Input: dimensioned drawing with shaded views. Units: mm. Origin: part minimum x, y, z. A direction names the side the tool comes from. Round coordinates to 2 decimals unless told otherwise and drop trailing zeros. Loops run counter-clockwise (first coordinate to the right, second up) from the corner with the lowest first, then second, coordinate; pieces in that order, holes last. Notation, with made-up numbers: M 50.5,59.5 L 106.5,59.5 A21 ccw 106.5,69.5 Z; hole C 2,41 d4. An arc over 180 degrees is marked long. One line per item, written item: value.
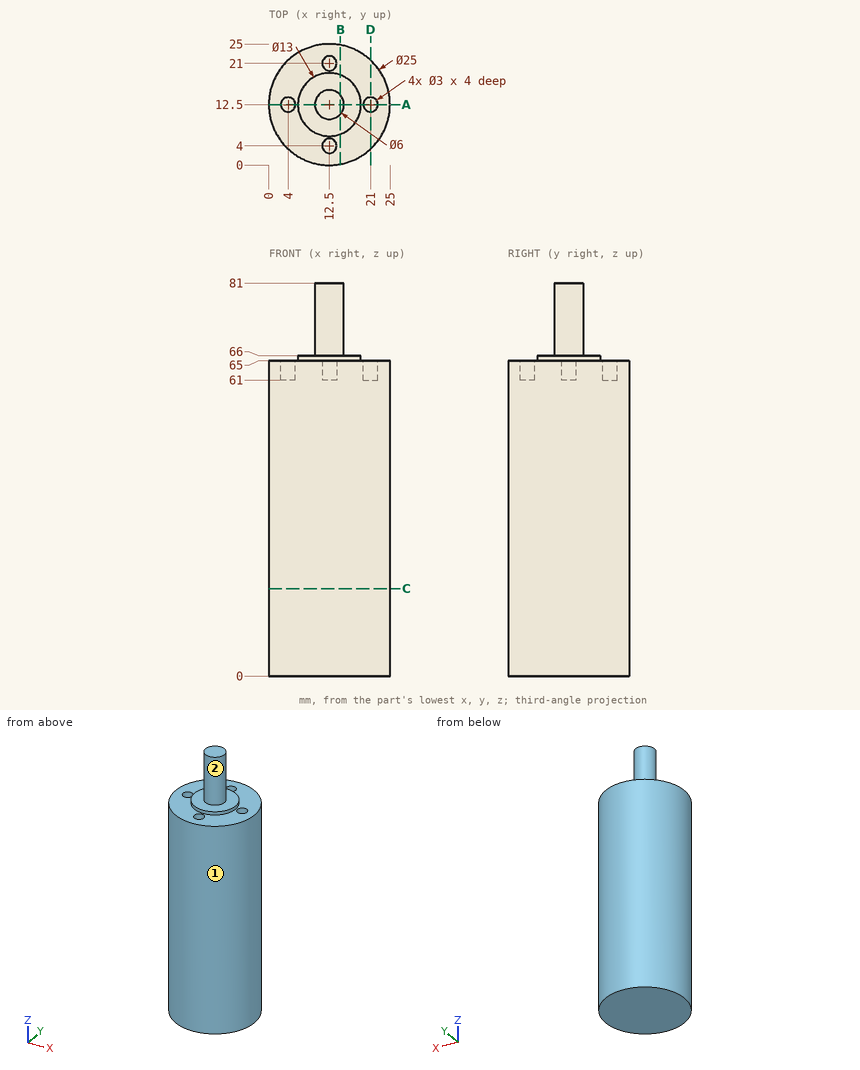
1. Section query D-D (x = 21). Return the cut outline in (y, z).
Report:
outline: M 3.33,0 L 21.67,0 L 21.67,65 L 14,65 L 14,61 L 11,61 L 11,65 L 3.33,65 Z
2. Section query C-C (z = 18). Return the cut outline in (x, y), and give its area (3 significant figures).
Report:
outline: C 12.5,12.5 d25
area: 491 mm2
3. Reachability of the marked faces 1 and 2 from +Z, -Z, +X, -X, +Y, -Y: full face, straight path, thin tool, end or side. Return the list, or none.
Report:
face 1: +Z, -Z
face 2: +Z
4. Section query A-A (y = 12.5). Return the cut outline in (x, z).
Report:
outline: M 0,0 L 25,0 L 25,65 L 22.5,65 L 22.5,61 L 19.5,61 L 19.5,65 L 19,65 L 19,66 L 15.5,66 L 15.5,81 L 9.5,81 L 9.5,66 L 6,66 L 6,65 L 5.5,65 L 5.5,61 L 2.5,61 L 2.5,65 L 0,65 Z
5. Pin query (flat end, axial travel): pin 1 (3 mm diameter, centred on x = 16, y = 7.5, fed in from +Z); pin 2 (3.5 mm diameter, centred on x = 12, y = 21.5, fed in from +Z); pin 3 (1 mm diameter, centred on y = 9, z = 61, fed in from -X). Return the tip coordinate at first contact, or that it passes through.
Report:
pin 1: stops at z = 66
pin 2: stops at z = 65
pin 3: stops at x = 0.37
6. Ray query, line 1 (Y direction, x = 12.5, z = 62.7); line 2 (Z direction, x = 17, y = 8.5); line 3 (Z direction, x = 3.5, y = 10.75). Return the intervals inside material, ascending. Write a range as [from, to].
Report:
line 1: y = [0, 2.5], [5.5, 19.5], [22.5, 25]
line 2: z = [0, 66]
line 3: z = [0, 65]
7. Section query B-B (x = 14.75). Return the cut outline in (y, z), and give its area (3 significant figures).
Report:
outline: M 0.2,0 L 24.8,0 L 24.8,65 L 18.6,65 L 18.6,66 L 14.48,66 L 14.48,81 L 10.52,81 L 10.52,66 L 6.4,66 L 6.4,65 L 0.2,65 Z
area: 1,670 mm2
